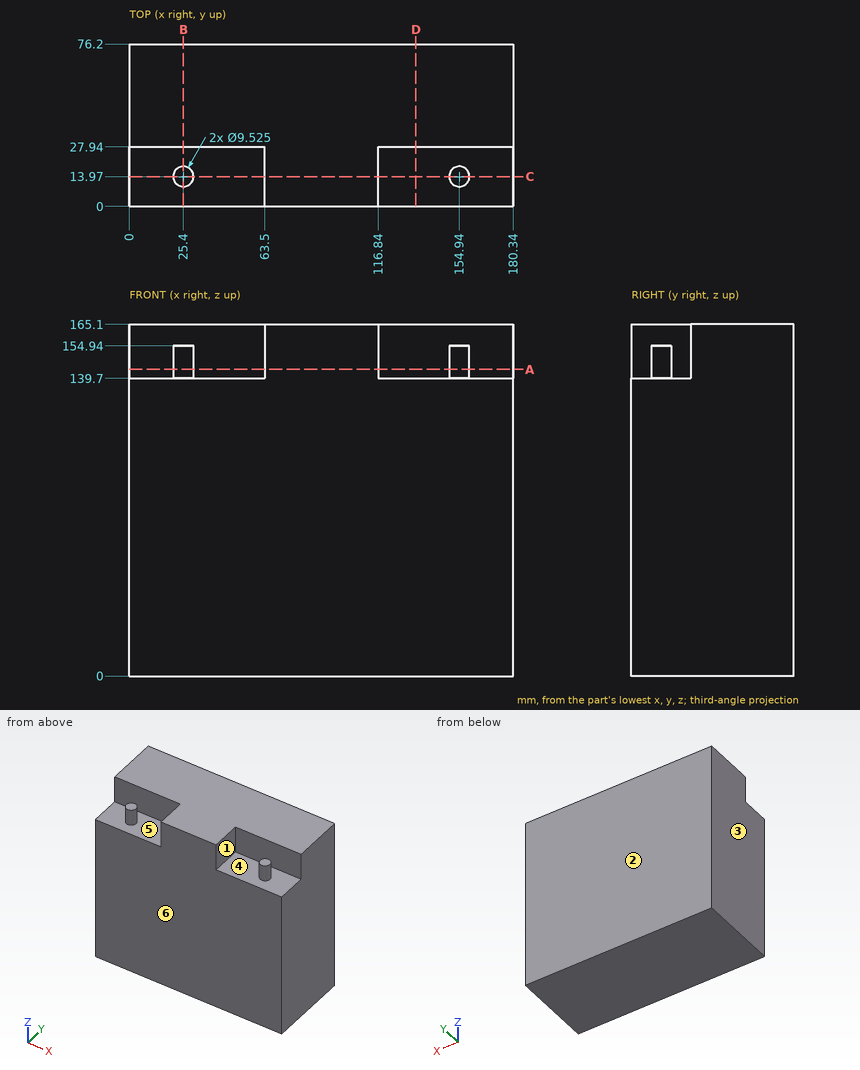
Design review of the part shown in the three views and the two pictorial views. Dimensions are in mm from the part's minimum x, y and z. A direction names the side the tool comes from. Round coordinates to 2 decimals unless told otherwise and drop trailing zeros. Write each loop counter-clockwise with the first axis right and the second up, starting at its lowest first coordinate (ties: lowest second). Pieces come first, ordered by that corner, then holes.
Item 1: Consider section C-C on y = 13.97. Give the boundary of the cut face in (x, z), and give its area (3 significant figures).
Item 2: For pin 1 Ø12.5 at (y, z) = (20.5, 153.5) entering from -X; pin 2 Ø10.5 at (x, y) = (23, 13.5) entering from +Z; pin 3 Ø12.5 at (x, z) = (29.5, 152.5) entering from -Y, all flat-tipped, find the tip position at first contact; note any pin that passes through.
Item 3: Consider section D-D on x = 134.5. Give the boundary of the cut face in (y, z).
Item 4: Consider section B-B on x = 25.4. Give the boundary of the cut face in (y, z), and give its area (3 significant figures).
Item 5: For the marked faces 1 and 2, list the 3-axis set-ups (+Z, -Z, +X, -X, +Y, -Y) from which the entire face can be reached by the end or side of a thin tool; tool diameter is ignored.
Item 6: Consider section A-A on z = 144. Give the boundary of the cut face in (x, y) (1 decimal), and give its area (3 significant figures).
Item 7: Wall thickness on L1, parallel to Z at x = 25, y = 25; L2, parallel to Y at x = 39.5, z = 142; L3, parallel to Z at x = 154, y = 17: over which ranges is each line inside the solid? List them lowest first.
Item 8: Draft analysis for pull direction X (two halves, no side actions). For the marked faces 3, 4, 5 and 6, state which applies: released by +X, released by -X, zero draft, split by the parting line, or undercut.
Check values:
1. outline: (0, 0) - (180.34, 0) - (180.34, 139.7) - (159.7, 139.7) - (159.7, 154.94) - (150.18, 154.94) - (150.18, 139.7) - (116.84, 139.7) - (116.84, 165.1) - (63.5, 165.1) - (63.5, 139.7) - (30.16, 139.7) - (30.16, 154.94) - (20.64, 154.94) - (20.64, 139.7) - (0, 139.7) - close
1. area: 26,800 mm2
2. pin 1: stops at x = 20.65
2. pin 2: stops at z = 154.94
2. pin 3: stops at y = 9.21
3. outline: (0, 0) - (76.2, 0) - (76.2, 165.1) - (27.94, 165.1) - (27.94, 139.7) - (0, 139.7) - close
4. outline: (0, 0) - (76.2, 0) - (76.2, 165.1) - (27.94, 165.1) - (27.94, 139.7) - (18.73, 139.7) - (18.73, 154.94) - (9.21, 154.94) - (9.21, 139.7) - (0, 139.7) - close
4. area: 12,000 mm2
5. face 1: +Z, -Y
5. face 2: +Z, -Z, +X, -X, +Y
6. outline: (0, 27.9) - (63.5, 27.9) - (63.5, 0) - (116.8, 0) - (116.8, 27.9) - (180.3, 27.9) - (180.3, 76.2) - (0, 76.2) - close; circle Ø9.5 at (25.4, 14); circle Ø9.5 at (154.9, 14)
6. area: 10,300 mm2
7. L1: z = 0 to 139.7
7. L2: y = 27.94 to 76.2
7. L3: z = 0 to 154.94
8. face 3: released by -X
8. face 4: undercut
8. face 5: undercut
8. face 6: zero draft
